```python
from build123d import *

# Parameters (mm, degrees)
F1_DEPTH      = 40
F4_D          = 8.5
F4_DEPTH      = 100
F4_TIP        = 2.5536576309
F5_R          = 55
F6_DEPTH      = 100
F6_DEPTH_BACK = 400
F7_R          = 52.5
F8_DEPTH      = 480
F9_D          = 8.5
F9_DEPTH      = 30
F9_TIP        = 2.5536576309
F10_D         = 8.5
F10_DEPTH     = 30
F10_TIP       = 2.5536576309


with BuildPart() as f1:
    # F0 (on Front) → F1 (new body)
    with BuildSketch(Plane.XZ):
        Polygon((-199, 0), (0, 0), (0, 5), (-300, 5), (-300, 0), (-200, 0), (-268.9439998807, -57.8508848718), (-230.3767432995, -103.8135514589), (-225.9596969951, -100.107209534), (-261.3130155278, -57.9747651624), (-200.0294600783, -6.5517563875), (-164.6761415456, -48.6842007591), (-160.84591933, -45.4702627106), align=None)
    extrude(amount=F1_DEPTH)

    # F4
    with Locations(Plane(origin=(-186.3088176474, 0, -156.331660173), x_dir=(0, -1, 0), z_dir=(-0.7660444431, 0, -0.6427876097))):
        with Locations((20, 78.5575219373)):
            Hole(F4_D / 2, depth=F4_DEPTH)
            with Locations((0, 0, -(F4_DEPTH + F4_TIP / 2))):  # 118° drill point
                Cone(0, F4_D / 2, F4_TIP, mode=Mode.SUBTRACT)

    # F5 (on Right) → F6 (join, two sides)
    with BuildSketch(Plane.YZ) as f6_sk:
        with Locations((-20, 59.5)):
            Circle(F5_R)
    extrude(amount=F6_DEPTH)
    extrude(f6_sk.sketch, amount=-F6_DEPTH_BACK)

    # F7 (on face) → F8 (cut)
    with BuildSketch(Plane(origin=(-400, 0, 0), x_dir=(0, -1, 0), z_dir=(-1, 0, 0))):
        with Locations((20, 59.5)):
            Circle(F7_R)
    extrude(amount=-F8_DEPTH, mode=Mode.SUBTRACT)

    # F9 (one way)
    with BuildSketch(Plane.XY.offset(5)):
        with Locations((-280, -20), (-20, -20)):
            Circle(F9_D / 2)
    extrude(amount=-F9_DEPTH, mode=Mode.SUBTRACT)
    with Locations(Plane.XY.offset(5)):
        with Locations((-280, -20), (-20, -20)):
            with Locations((0, 0, -(F9_DEPTH + F9_TIP / 2))):  # 118° drill point
                Cone(0, F9_D / 2, F9_TIP, mode=Mode.SUBTRACT)

    # F10
    with Locations(Plane(origin=(0, 0, 5), x_dir=(1, 0, 0), z_dir=(0, 0, -1))):
        with Locations((-280, 20), (-20, 20)):
            Hole(F10_D / 2, depth=F10_DEPTH)
            with Locations((0, 0, -(F10_DEPTH + F10_TIP / 2))):  # 118° drill point
                Cone(0, F10_D / 2, F10_TIP, mode=Mode.SUBTRACT)


solid = f1.part
```
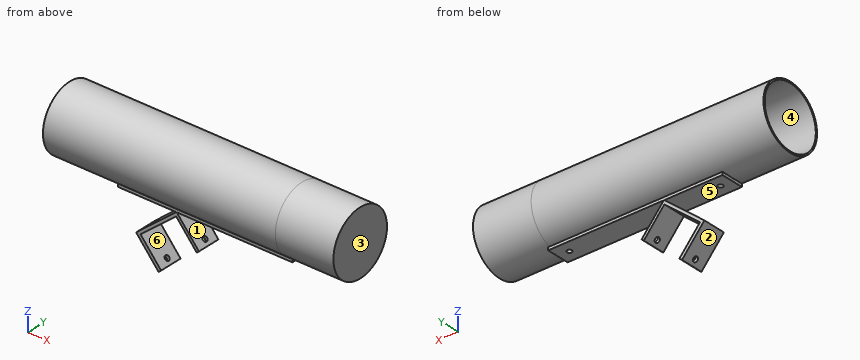
Verification items for the finished model (mm, model axes). Face numbers are marked on the shaded views. A direction names the side the tool comes from. Coordinates: 2 decimals unless noted, no trailing zeros. Loops run counter-clockwise (first coordinate to the right, second up) from the corner with the lowest first, then second, coordinate; pieces in that order, holes last. Notation, with made-up numbers: (23, 72.25) -> (35, 72.25) arc R27 ccw to (35, 105.25) -> close; hole circle Ø2 at (16, 16). An arc over 180 degrees is marked (long way). Put each result on its own line as item: value.
1. Gauge pin test, flat ends, axial feed: P1, Ø4, axis at x = -247.5, y = -26, coming from the -Z side; P2, Ø8, axis at x = -0.5, z = 7.5, coming from the +Y side; P3, Ø12, axis at x = -70, z = 37, coming from the -Y side. Record the tip position at first contact, or that the pin passes through.
Result set:
P1: stops at z = -85.79
P2: stops at y = 6.85
P3: stops at y = -72.47
2. Section check A-A, the plane x = -245. Record the boundary of the cut face in (y, z), then the cut area to 3 significant figures.
Result set:
outline: (-40, -86.39) -> (0, -86.39) -> (0, -77.42) -> (-40, -77.42) -> close; (-40, -44.29) -> (0, -44.29) -> (0, -37.76) -> (-40, -37.76) -> close; (-40, 0) -> (0, 0) -> (0, 5) -> (-12.6, 5) arc R55 ccw (long way) to (-27.4, 5) -> (-40, 5) -> close; hole circle Ø105 at (-20, 59.5)
area: 1,660 mm^2
3. Thickness scan on line 1 (X direction, y = -20, z = 5.8); line 2 (Z direction, x = 25, y = -22); line 3 (Z direction, x = -210, y = -20). Record the ranges inside material, lowest first.
Result set:
line 1: x = -400 to -284.25, -275.75 to -24.25, -15.75 to 100
line 2: z = 4.54 to 7.04, 111.96 to 114.46
line 3: z = -14.92 to -8.39, 0 to 7, 112 to 114.5
4. Section check D-D, the plane x = 63. Record the boundary of the cut face in (y, z), then the cut area to 3 significant figures.
Result set:
outline: circle Ø110 at (-20, 59.5); hole circle Ø105 at (-20, 59.5)
area: 844 mm^2
5. Section check B-B, the plane z = -15. Record the boundary of the cut face in (x, y).
Result set:
outline: (-217.88, -40) -> (-210.1, -40) -> (-210.1, 0) -> (-217.88, 0) -> close; (-192.94, -40) -> (-186.41, -40) -> (-186.41, 0) -> (-192.94, 0) -> close
6. Mould release check, pull along Z, two halves, no side actions. Record for the marked faces 1, 2 and 3: pulls with the +Z half, pulls with the -Z half, needs draft (parallel to the pull), parting line crosses it, or undercut.
Result set:
face 1: undercut
face 2: pulls with the -Z half
face 3: needs draft
7. Section check C-C, the plane y = 11.5. Record the boundary of the cut face in (x, z).
Result set:
outline: (-400, 14.41) -> (100, 14.41) -> (100, 104.59) -> (-400, 104.59) -> (-400, 101.5) -> (80, 101.5) -> (80, 17.5) -> (-400, 17.5) -> close
8. Tool access check on the marked faces 4, 5 and 6. Record the directions out of +Z, -Z, +X, -X, +Y, -Y that give a thin tool (end or side, any length) a straight path to the whole face; none if there is none.
Result set:
face 4: -X
face 5: -X, +Y, -Y
face 6: +X, +Y, -Y
